Input: part model. Units: mm. Frame: model coordinates. A direction names the side the tool comes from. Coordinates: 2 decimals unless noted, no trailing zeros. Order: outer loops, then holes, each group sorted by start corner. A loop starts at its lowest first (then second) coordinate and runs counter-clockwise, first axis right, second up. Notation, with made-up numbers: M -31,61.5 L 17,61.5 A28 cw 17,94.5 Z; hole C 1.25,43 d3. An arc over 180 degrees is marked long. Answer in a Markdown table with one row per item.
from build123d import *

# Parameters (mm, degrees)
SKETCH_1_W          = 19
SKETCH_1_H          = 26
EXTRUDE_1_DEPTH     = 3
CUT_EXTRUDE_START   = 3
SKETCH_1_3_R        = 3.05
SKETCH_1_3_R_2      = 1.05
CUT_EXTRUDE_1_DEPTH = 2.5
SKETCH_2_R          = 1
CUT_EXTRUDE_2_DEPTH = 1.5
SKETCH_2_3_R        = 0.7
CUT_EXTRUDE_3_DEPTH = 21.736441353
EXTRUDE_START       = 3
SKETCH_1_6_R        = 2
EXTRUDE_2_DEPTH     = 4
CUT_EXTRUDE_START_2 = 7
SKETCH_1_7_R        = 1.05
CUT_EXTRUDE_5_DEPTH = 4
SKETCH_3_R          = 0.3
CUT_EXTRUDE_6_DEPTH = 1.5


with BuildPart() as part:
    # 草图1 → 凸台-拉伸1 (new body)
    with BuildSketch(Plane(origin=(0, 0, 0), x_dir=(1, 0, 0), z_dir=(0, 1, 0))):
        with Locations((-4.5, -2)):
            Rectangle(SKETCH_1_W, SKETCH_1_H)
    extrude(amount=EXTRUDE_1_DEPTH)

    # 草图1<3> → 切除-拉伸1 (cut)
    with BuildSketch(Plane(origin=(0, 0, 0), x_dir=(1, 0, 0), z_dir=(0, 1, 0)).offset(CUT_EXTRUDE_START)):
        with Locations(Location((0, 0, 0), (0, 0, 90))):
            Circle(SKETCH_1_3_R)
        with Locations(Location((-8.107149516, 2.554237014, 0), (0, 0, 90))):
            Circle(SKETCH_1_3_R_2)
    extrude(amount=-CUT_EXTRUDE_1_DEPTH, mode=Mode.SUBTRACT)

    # 草图2 → 切除-拉伸2 (cut)
    with BuildSketch(Plane.XZ):
        with Locations(Location((-11.5, 12.5, 0), (0, 0, 270))):
            Circle(SKETCH_2_R)
        with Locations(Location((3, 6, 0), (0, 0, 270))):
            Circle(SKETCH_2_R)
    extrude(amount=-CUT_EXTRUDE_2_DEPTH, mode=Mode.SUBTRACT)

    # 草图2<3> → 切除-拉伸3 (cut, through all)
    with BuildSketch(Plane.XZ):
        with Locations(Location((-11.5, 12.5, 0), (0, 0, 270))):
            Circle(SKETCH_2_3_R)
        with Locations(Location((3, 6, 0), (0, 0, 270))):
            Circle(SKETCH_2_3_R)
    extrude(amount=-CUT_EXTRUDE_3_DEPTH, mode=Mode.SUBTRACT)

    # 草图1<6> → 凸台-拉伸2 (add)
    with BuildSketch(Plane(origin=(0, 0, 0), x_dir=(1, 0, 0), z_dir=(0, 1, 0)).offset(EXTRUDE_START)):
        with Locations(Location((-8.107149516, 2.554237014, 0), (0, 0, 90))):
            Circle(SKETCH_1_6_R)
    extrude(amount=EXTRUDE_2_DEPTH)

    # 草图1<7> → 切除-拉伸5 (cut)
    with BuildSketch(Plane(origin=(0, 0, 0), x_dir=(1, 0, 0), z_dir=(0, 1, 0)).offset(CUT_EXTRUDE_START_2)):
        with Locations(Location((-8.107149516, 2.554237014, 0), (0, 0, 90))):
            Circle(SKETCH_1_7_R)
    extrude(amount=-CUT_EXTRUDE_5_DEPTH, mode=Mode.SUBTRACT)

    # 草图3 → 切除-拉伸6 (cut)
    with BuildSketch(Plane.XY.offset(-11)):
        with Locations((0.8, 1.5)):
            Circle(SKETCH_3_R)
        with Locations((-4.2, 1.5)):
            Circle(SKETCH_3_R)
    extrude(amount=CUT_EXTRUDE_6_DEPTH, mode=Mode.SUBTRACT)


solid = part.part
1) Contact query for flat-ended pins moving along their axis: pin 1 (1.8 mm diameter, centred on x = 3, z = 6, fed in from -Y); pin 2 (1.8 mm diameter, centred on x = -11.5, z = 12.5, fed in from +Y); pin 3 (4 mm diameter, centred on x = 1, y = 6, fed in from +Z). Output: stop coordinate, or through.
Resolved:
| item | result |
|---|---|
| pin 1 | stops at y = 1.5 |
| pin 2 | stops at y = 3 |
| pin 3 | passes through |
2) Material intervals for probe 1 along Y at (x, z) = (0.8, -10.1); probe 2 along X at (y, z) = (2.4, 12.5); probe 3 along Y at (x, z) = (-11, 7), sorted ascending.
Resolved:
| item | result |
|---|---|
| probe 1 | y = 0 to 1.2, 1.8 to 3 |
| probe 2 | x = -14 to -12.2, -10.8 to 5 |
| probe 3 | y = 0 to 3 |
3) Cut plane D-D, the plane z = -6.5. Output: boundary loops of the cut face in (x, y).
Resolved:
| item | result |
|---|---|
| outline | M -14,0 L 5,0 L 5,3 L -14,3 Z |
4) Reachability of faces 1 (the face through (-7.08, 3.8, -2.33)), 2 (the face through (3, 2.2, 6.7)), 3 (the face through (-10.51, 0.74, 12.63)) from +Z, -Z, +X, -X, +Y, -Y: full face, straight path, thin tool, end or side. Return the list, or none.
Resolved:
| item | result |
|---|---|
| face 1 | +Y |
| face 2 | +Y, -Y |
| face 3 | -Y |
5) Cut plane A-A, the plane z = 6. Output: boundary loops of the cut face in (x, y), and give its area (3 significant figures).
Resolved:
| item | result |
|---|---|
| outline | M -14,0 L 2,0 L 2,1.5 L 2.3,1.5 L 2.3,3 L -14,3 Z; M 3.7,1.5 L 4,1.5 L 4,0 L 5,0 L 5,3 L 3.7,3 Z |
| area | 51.9 mm2 |
6) Mould query, pull axis X, two halves, no side actions, for faces 4 (the face through (-10.09, 4.97, -2.29)), 5 (the face through (-5, 1, -11)), 6 (the face through (3.676, 0.74, 6.737)). Classes: +X half, -X half, draft (parallel to the pull), parting line (faces both ways), or undercut.
Resolved:
| item | result |
|---|---|
| face 4 | parting line |
| face 5 | draft |
| face 6 | undercut |
7) Cut plane B-B, the plane x = -4.2. Output: boundary loops of the cut face in (y, z).
Resolved:
| item | result |
|---|---|
| outline | M 0,-11 L 1.2,-11 L 1.2,-9.5 L 1.8,-9.5 L 1.8,-11 L 3,-11 L 3,15 L 0,15 Z |
8) Cut plane C-C, the plane y = 2.5. Output: boundary loops of the cut face in (x, z).
Resolved:
| item | result |
|---|---|
| outline | M -14,-11 L 5,-11 L 5,15 L -14,15 Z; hole C -11.5,12.5 d1.4; hole C -8.11,-2.55 d2.1; hole C 0,0 d6.1; hole C 3,6 d1.4 |
